Design review of the part built by this model. Coordinates are the model's own, in mm. A direction names the side the tool comes from. Coordinates: 2 decimals unless noted, no trailing zeros. Order: outer loops, then holes, each group sorted by start corner. A loop starts at its lowest first (then second) coordinate and runs counter-clockwise, first axis right, second up. Notation, with made-up numbers: M 33,34.5 L 54,34.5 A5 ccw 54,43.5 Z; hole C -32.75,-15 d5. An arc over 180 degrees is marked long. Use CSV: the item, a comma, the result in double quotes.
```python
from build123d import *

# Parameters (mm, degrees)
F1_DEPTH = 25
F2_R     = 3.5
F3_DEPTH = 25
F4_R     = 3


with BuildPart() as f1:
    # F0 (on Top) → F1 (new body)
    with BuildSketch(Plane.XY):
        with BuildLine():
            ThreePointArc((-8.2, 12.5602547745), (-7.1414284285, -13.1909059583), (15, 0))
            ThreePointArc((15, 0), (13.1909059583, 7.1414284285), (8.2, 12.5602547745))
            ThreePointArc((8.2, 12.5602547745), (5.3232312755, 14.0236660253), (2.2, 14.8377895928))
            Line((2.2, 14.8377895928), (2.2, 10.0091561408))
            ThreePointArc((2.2, 10.0091561408), (7.9865195614, 6.4217374554), (10.248083072, 0))
            ThreePointArc((10.248083072, 0), (-6.4217374554, -7.9865195614), (-2.2, 10.0091561408))
            Line((-2.2, 10.0091561408), (-2.2, 14.8377895928))
            ThreePointArc((-2.2, 14.8377895928), (-5.3232312755, 14.0236660253), (-8.2, 12.5602547745))
        make_face()
        with BuildLine():
            Line((-8.2, 25.4279577023), (-8.2, 12.5602547745))
            ThreePointArc((-8.2, 12.5602547745), (-5.3232312755, 14.0236660253), (-2.2, 14.8377895928))
            Line((-2.2, 14.8377895928), (-2.2, 25.4279577023))
            Line((-2.2, 25.4279577023), (-8.2, 25.4279577023))
        make_face()
        with BuildLine():
            ThreePointArc((2.2, 14.8377895928), (5.3232312755, 14.0236660253), (8.2, 12.5602547745))
            Line((8.2, 12.5602547745), (8.2, 25.4279577023))
            Line((8.2, 25.4279577023), (2.2, 25.4279577023))
            Line((2.2, 25.4279577023), (2.2, 14.8377895928))
        make_face()
    extrude(amount=F1_DEPTH)

    # F2 (on face) → F3 (cut)
    with BuildSketch(Plane.YZ.offset(8.2)):
        with Locations((18.9941062384, 12.5)):
            Circle(F2_R)
    extrude(amount=-F3_DEPTH, mode=Mode.SUBTRACT)

    # F4
    f4_edges = [f1.edges().sort_by_distance(p)[0] for p in [
        (8.2, 12.560255, 12.5),
        (-8.2, 12.560255, 12.5),
    ]]
    fillet(f4_edges, radius=F4_R)


solid = f1.part
```
(1) The part is to be moulded in two halves that separate along Y. For faces 1 (the face through (-2.2, 16, 10)), 2 (the face through (8.506, 12.77, 12.675)), 3 (the face through (5.242, 22.227, 11.159)), 4 (the face through (-5.158, 22.227, 11.159)), say which applies: pulls with the +Y half, pulls with the -Y half, needs draft (parallel to the pull), parting line crosses it, or undercut.
The answers:
face 1,"needs draft"
face 2,"pulls with the +Y half"
face 3,"undercut"
face 4,"undercut"
(2) Add section B-B on y = 0. State the section outline as (x, z) points, and give its area (3 significant figures).
The answers:
outline,"M -15,0 L -10.25,0 L -10.25,25 L -15,25 Z; M 10.25,0 L 15,0 L 15,25 L 10.25,25 Z"
area,"238 mm2"
(3) Add section C-C on z = 11.5. State the section outline as (x, y) points, and give its area (3 significant figures).
The answers:
outline,"M -9.33,11.74 A15 ccw long 9.33,11.74 A3 cw 8.2,14.09 L 8.2,15.64 L 2.2,15.64 L 2.2,10.01 A10.25 cw long -2.2,10.01 L -2.2,15.64 L -8.2,15.64 L -8.2,14.09 A3 cw Z; M -8.2,22.35 L -2.2,22.35 L -2.2,25.43 L -8.2,25.43 Z; M 2.2,22.35 L 8.2,22.35 L 8.2,25.43 L 2.2,25.43 Z"
area,"414 mm2"
(4) Wall thickness on probe 1 along Y at (x, z) = (5, 11.5); probe 2 along X at (y, z) = (0, 12.5); probe 3 along Y at (x, z) = (4, 10): over which ranges is each line inside the solid? List them lowest first.
The answers:
probe 1,"y = -14.14 to -8.95, 8.95 to 15.64, 22.35 to 25.43"
probe 2,"x = -15 to -10.25, 10.25 to 15"
probe 3,"y = -14.46 to -9.44, 9.44 to 16.54, 21.44 to 25.43"
(5) Add section D-D on z = 18.5. State the section outline as (x, y) points.
The answers:
outline,"M -9.33,11.74 A15 ccw long 9.33,11.74 A3 cw 8.2,14.09 L 8.2,25.43 L 2.2,25.43 L 2.2,10.01 A10.25 cw long -2.2,10.01 L -2.2,25.43 L -8.2,25.43 L -8.2,14.09 A3 cw Z"
(6) Add section A-A on x = 4. State the section outline as (y, z) points, and give its area (3 significant figures).
The answers:
outline,"M -14.46,0 L -9.44,0 L -9.44,25 L -14.46,25 Z; M 9.44,0 L 25.43,0 L 25.43,25 L 9.44,25 Z; hole C 18.99,12.5 d7"
area,"487 mm2"
(7) Clearance check with flat-ended pins moving along their axes: P1, Ø1.5, axis at y = 18, z = 11, coming from the -X side; P2, Ø10, axis at y = 9, z = 2.5, coming from the +X side; P3, Ø12.5, axis at y = 20.5, z = 17, coming from the +X side; P4, Ø10, axis at y = -6.5, z = 3, coming from the +X side. State where each tip first meets the part, or that it passes through.
The answers:
P1,"passes through"
P2,"stops at x = 14.46"
P3,"stops at x = 8.2"
P4,"stops at x = 14.92"
(8) For faces 5 (the face through (2.2, 16, 10)), 6 (the face through (-4, 10, 0)), 7 (the face through (8.2, 22, 10)), 8 (the face through (-8.2, 21.1, 9.5)), list the 3-axis set-ups (+Z, -Z, +X, -X, +Y, -Y) from which the entire face can be reached by the end or side of a thin tool; tool diameter is ignored.
The answers:
face 5,"+Z, -Z, +Y"
face 6,"-Z, +X, -X, +Y, -Y"
face 7,"+Z, -Z, +X, +Y"
face 8,"+Z, -Z, -X, +Y"
